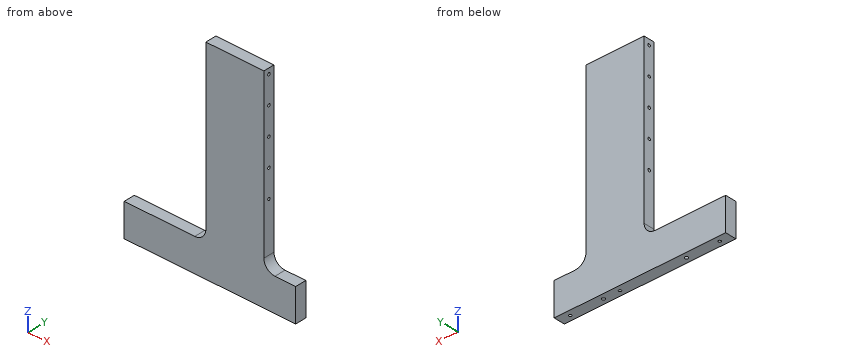
```python
from build123d import *

# Parameters (mm, degrees)
AUFSATZ_LINEAR_AUSTRAGEN1_DEPTH       = 20
M6_GEWINDEBOHRUNG1_AT_2_COUNT         = 2
M6_GEWINDEBOHRUNG1_AT_2_PITCH         = 50
M6_GEWINDEBOHRUNG1_AT_3_COUNT         = 2
M6_GEWINDEBOHRUNG1_AT_3_PITCH         = 100
M6_GEWINDEBOHRUNG1_AT_4_COUNT         = 2
M6_GEWINDEBOHRUNG1_AT_4_PITCH         = 150
M6_GEWINDEBOHRUNG1_AT_5_COUNT         = 2
M6_GEWINDEBOHRUNG1_AT_5_PITCH         = 206.155281281
M6_GEWINDEBOHRUNG1_AT_6_COUNT         = 2
M6_GEWINDEBOHRUNG1_AT_6_PITCH         = 200
M6_GEWINDEBOHRUNG2_D                  = 5
M6_GEWINDEBOHRUNG2_DEPTH              = 17
M6_GEWINDEBOHRUNG2_TIP                = 1.502151548
VERRUNDUNG1_R                         = 20
F_6_0MM_TRANSITIONAL_STIFTLOCH1_D     = 6
F_6_0MM_TRANSITIONAL_STIFTLOCH1_DEPTH = 17
F_6_0MM_TRANSITIONAL_STIFTLOCH1_TIP   = 1.802581857


with BuildPart() as part:
    # Skizze1 → Aufsatz-Linear austragen1 (new body)
    with BuildSketch(Plane(origin=(0, 0, 0), x_dir=(1, 0, 0), z_dir=(0, 1, 0))):
        Polygon((-52.5, 0), (52.5, 0), (52.5, 320), (110, 320), (110, 380), (-200, 380), (-200, 320), (-52.5, 320), align=None)
    extrude(amount=AUFSATZ_LINEAR_AUSTRAGEN1_DEPTH)

    # Skizze4 → M6 Gewindebohrung1 (revolve, cut)
    with BuildSketch(Plane(origin=(52.5, 10, -10), x_dir=(0, 0, -1), z_dir=(0, 1, 0))):
        Polygon((0, 0), (0, 18.502151548), (2.5, 17), (2.5, 0), align=None)
    m6_gewindebohrung1 = revolve(axis=Axis((58.85, 10, -10), (-1, 0, 0)), mode=Mode.SUBTRACT)

    # M6 Gewindebohrung1 at 2: M6 Gewindebohrung1 ×2
    with Locations(*[(0, 0, -i * M6_GEWINDEBOHRUNG1_AT_2_PITCH) for i in range(1, M6_GEWINDEBOHRUNG1_AT_2_COUNT)]):
        add(m6_gewindebohrung1, mode=Mode.SUBTRACT)

    # M6 Gewindebohrung1 at 3: M6 Gewindebohrung1 ×2
    with Locations(*[(0, 0, -i * M6_GEWINDEBOHRUNG1_AT_3_PITCH) for i in range(1, M6_GEWINDEBOHRUNG1_AT_3_COUNT)]):
        add(m6_gewindebohrung1, mode=Mode.SUBTRACT)

    # M6 Gewindebohrung1 at 4: M6 Gewindebohrung1 ×2
    with Locations(*[(0, 0, -i * M6_GEWINDEBOHRUNG1_AT_4_PITCH) for i in range(1, M6_GEWINDEBOHRUNG1_AT_4_COUNT)]):
        add(m6_gewindebohrung1, mode=Mode.SUBTRACT)

    # M6 Gewindebohrung1 at 5: M6 Gewindebohrung1 ×2
    with Locations(*[Vector(0, 0.242535625, -0.9701425) * (i * M6_GEWINDEBOHRUNG1_AT_5_PITCH) for i in range(1, M6_GEWINDEBOHRUNG1_AT_5_COUNT)]):
        add(m6_gewindebohrung1, mode=Mode.SUBTRACT)

    # M6 Gewindebohrung1 at 6: M6 Gewindebohrung1 ×2
    with Locations(*[(0, 0, -i * M6_GEWINDEBOHRUNG1_AT_6_PITCH) for i in range(1, M6_GEWINDEBOHRUNG1_AT_6_COUNT)]):
        add(m6_gewindebohrung1, mode=Mode.SUBTRACT)

    # Spiegeln1: M6 Gewindebohrung1 across plane
    add(m6_gewindebohrung1.mirror(Plane(origin=(0, 0, 0), x_dir=(0, 0, 1), z_dir=(1, 0, 0))), mode=Mode.SUBTRACT)

    # Spiegeln1 copy 1 sketch → Spiegeln1 copy 1 (revolve, cut)
    with BuildSketch(Plane(origin=(-52.5, 10, -60), x_dir=(0, 0, -1), z_dir=(0, 1, 0))):
        Polygon((0, 0), (0, -18.502151548), (2.5, -17), (2.5, 0), align=None)
    revolve(axis=Axis((-58.85, 10, -60), (-1, 0, 0)), mode=Mode.SUBTRACT)

    # Spiegeln1 copy 2 sketch → Spiegeln1 copy 2 (revolve, cut)
    with BuildSketch(Plane(origin=(-52.5, 10, -110), x_dir=(0, 0, -1), z_dir=(0, 1, 0))):
        Polygon((0, 0), (0, -18.502151548), (2.5, -17), (2.5, 0), align=None)
    revolve(axis=Axis((-58.85, 10, -110), (-1, 0, 0)), mode=Mode.SUBTRACT)

    # Spiegeln1 copy 3 sketch → Spiegeln1 copy 3 (revolve, cut)
    with BuildSketch(Plane(origin=(-52.5, 10, -160), x_dir=(0, 0, -1), z_dir=(0, 1, 0))):
        Polygon((0, 0), (0, -18.502151548), (2.5, -17), (2.5, 0), align=None)
    revolve(axis=Axis((-58.85, 10, -160), (-1, 0, 0)), mode=Mode.SUBTRACT)

    # Spiegeln1 copy 4 sketch → Spiegeln1 copy 4 (revolve, cut)
    with BuildSketch(Plane(origin=(-52.5, 60, -210), x_dir=(0, 0, -1), z_dir=(0, 1, 0))):
        Polygon((0, 0), (0, -18.502151548), (2.5, -17), (2.5, 0), align=None)
    revolve(axis=Axis((-58.85, 60, -210), (-1, 0, 0)), mode=Mode.SUBTRACT)

    # Spiegeln1 copy 5 sketch → Spiegeln1 copy 5 (revolve, cut)
    with BuildSketch(Plane(origin=(-52.5, 10, -210), x_dir=(0, 0, -1), z_dir=(0, 1, 0))):
        Polygon((0, 0), (0, -18.502151548), (2.5, -17), (2.5, 0), align=None)
    revolve(axis=Axis((-58.85, 10, -210), (-1, 0, 0)), mode=Mode.SUBTRACT)

    # M6 Gewindebohrung2
    with Locations(Plane(origin=(0, 0, -380), x_dir=(-1, 0, 0), z_dir=(0, 0, -1))):
        with Locations((-90, 10), (180, 10), (0, 10)):
            Hole(M6_GEWINDEBOHRUNG2_D / 2, depth=M6_GEWINDEBOHRUNG2_DEPTH)
            with Locations((0, 0, -(M6_GEWINDEBOHRUNG2_DEPTH + M6_GEWINDEBOHRUNG2_TIP / 2))):  # 118° drill point
                Cone(0, M6_GEWINDEBOHRUNG2_D / 2, M6_GEWINDEBOHRUNG2_TIP, mode=Mode.SUBTRACT)

    # Verrundung1
    verrundung1_edges = [part.edges().sort_by_distance(p)[0] for p in [
        (-52.5, 10, -320),
        (52.5, 10, -320),
    ]]
    fillet(verrundung1_edges, radius=VERRUNDUNG1_R)

    # Ø6.0mm Transitional Stiftloch1
    with Locations(Plane(origin=(0, 0, -380), x_dir=(-1, 0, 0), z_dir=(0, 0, -1))):
        with Locations((120, 10), (-30, 10)):
            Hole(F_6_0MM_TRANSITIONAL_STIFTLOCH1_D / 2, depth=F_6_0MM_TRANSITIONAL_STIFTLOCH1_DEPTH)
            with Locations((0, 0, -(F_6_0MM_TRANSITIONAL_STIFTLOCH1_DEPTH + F_6_0MM_TRANSITIONAL_STIFTLOCH1_TIP / 2))):  # 118° drill point
                Cone(0, F_6_0MM_TRANSITIONAL_STIFTLOCH1_D / 2, F_6_0MM_TRANSITIONAL_STIFTLOCH1_TIP, mode=Mode.SUBTRACT)


solid = part.part
```
Geometry check sheet. Reference: the model listing, model coordinates, mm. Coordinates: 2 decimals unless noted, no trailing zeros. Write each loop counter-clockwise with the first axis right and the second up, starting at its lowest first coordinate (ties: lowest second). Pieces come first, ordered by that corner, then holes. Notation, with made-up numbers: (58.5, 20) -> (89.5, 20) arc R13 ccw to (89.5, 43) -> close; hole circle Ø1 at (53, 85.25). An arc over 180 degrees is marked (long way). Use CSV: the item, a comma, the result in double quotes. Start each with the question number.
Item 1: Cross-section at C-C, the plane x = 62. Record the cut outline in (y, z).
Item 2: Cross-section at A-A, the plane y = 16. Record the cut outline in (x, z), plus the area to 3 significant figures.
Item 3: Thickness scan on line 1 (Z direction, x = 45.25, y = 10); line 2 (Y direction, x = -45, z = -60); line 3 (X direction, y = 10, z = -369.75). Record the ranges inside material, lowest first.
Item 4: Depth check by flat-ended pin: pin 1 Ø10 at (y, z) = (11, -174) entering from -X; pin 2 Ø4 at (y, z) = (4.5, -60.5) entering from +X; pin 3 Ø4.5 at (y, z) = (10, -110) entering from -X; pin 4 Ø8 at (x, y) = (30, 10) entering from -Z. Enter the tip coordinate at first touch or a pass-through.
Item 5: Cross-section at B-B, the plane z = -220.5. Record the cut outline in (x, y).
Answers:
1,outline,"(0, -380) -> (20, -380) -> (20, -317.02) -> (0, -317.02) -> close"
2,outline,"(-200, -380) -> (110, -380) -> (110, -320) -> (72.5, -320) arc R20 cw to (52.5, -300) -> (52.5, 0) -> (-52.5, 0) -> (-52.5, -300) arc R20 cw to (-72.5, -320) -> (-200, -320) -> close"
2,area,"52,400 mm^2"
3,line 1,"-380 to -212.5, -207.5 to -162.5, -157.5 to -112.5, -107.5 to -62.5, -57.5 to -12.5, -7.5 to 0"
3,line 2,"0 to 7.5, 12.5 to 20"
3,line 3,"-200 to -182.5, -177.5 to -123, -117 to -2.5, 2.5 to 27, 33 to 87.5, 92.5 to 110"
4,pin 1,"x = -52.5"
4,pin 2,"x = 52.5"
4,pin 3,"x = -35.35"
4,pin 4,"z = -380"
5,outline,"(-52.5, 0) -> (52.5, 0) -> (52.5, 20) -> (-52.5, 20) -> close"
